from build123d import *

# Parameters (mm, degrees)
BO_ALTMA1_T                 = -1.5
KES_EKSTR_ZYON1_DEPTH       = 2
Y_KSEKLIK_EKSTR_ZYON4_DEPTH = 2
RADYUS1_R                   = 1.3
Y_KSEKLIK_EKSTR_ZYON5_DEPTH = 1.5
RADYUS2_R                   = 1
IZIM7_R                     = 2.75
KES_EKSTR_ZYON2_DEPTH       = 10
IZIM8_R                     = 1.5
KES_EKSTR_ZYON3_DEPTH       = 10
PAH1_SIZE                   = 1.656848502
PAH1_SIZE_2                 = 1.6


# Some blends are built 0.0001 mm under size
with BuildPart() as part:
    # Çizim3 → Loft4 section 0
    with BuildSketch(Plane(origin=(0, 20, 0), x_dir=(1, 0, 0), z_dir=(0, 1, 0))):
        with BuildLine():
            Line((-40, 18), (40, 18))
            Line((40, 18), (40, -18))
            Line((40, -18), (-40, -18))
            Line((-40, -18), (-40, 18))
        make_face()
    # Çizim1 → Loft4 section 1
    with BuildSketch(Plane(origin=(0, 0, 0), x_dir=(1, 0, 0), z_dir=(0, 1, 0))):
        with BuildLine():
            Line((-47.5, 25), (47.5, 25))
            Line((47.5, 25), (47.5, -25))
            Line((47.5, -25), (-47.5, -25))
            Line((-47.5, -25), (-47.5, 25))
        make_face()
    loft()

    # İç Boşaltma1
    bo_altma1_openings = [part.faces().sort_by_distance(p)[0] for p in [
        (0, 0, 0),
    ]]
    offset(amount=BO_ALTMA1_T, openings=bo_altma1_openings, kind=Kind.INTERSECTION)

    # Çizim4 → Kes-Ekstrüzyon1 (cut)
    with BuildSketch(Plane(origin=(0, 20, 0), x_dir=(1, 0, 0), z_dir=(0, 1, 0))):
        with BuildLine():
            Line((-17.459780383, 9.572622818), (-4.814835579, 9.572622818))
            ThreePointArc((-4.814835579, 9.572622818), (4.757787239, 0), (-4.814835579, -9.572622818))
            Line((-4.814835579, -9.572622818), (-17.459780383, -9.572622818))
            ThreePointArc((-17.459780383, -9.572622818), (-27.032403201, 0), (-17.459780383, 9.572622818))
        make_face()
    extrude(amount=-KES_EKSTR_ZYON1_DEPTH, mode=Mode.SUBTRACT)

    # Çizim5 → Yükseklik-Ekstrüzyon4 (add)
    with BuildSketch(Plane(origin=(0, 7.299574586, -20.855927387), x_dir=(1, 0, 0), z_dir=(0, -0.33035042472810616, 0.9438583563660173))):
        Polygon((-21.117307497, 9.666637975), (-39.739182442, 9.666637975), (-40.270102767, 8.166637975), (-21.117307497, 8.166637975), align=None)
    extrude(amount=Y_KSEKLIK_EKSTR_ZYON4_DEPTH)

    # Radyus1
    # the kernel refuses this fillet: 1.3 mm, written as the material it takes off along each edge
    with BuildSketch(Plane(origin=(-43.520102767, 14.347023232, -16.270358351), x_dir=(0, 0.3303504247281054, -0.9438583563660177), z_dir=(1, 0, 0))) as radyus1_piece_1_section:
        with BuildLine():
            CenterArc((RADYUS1_R, RADYUS1_R), RADYUS1_R, 180, 90)
            Line((0, RADYUS1_R), (0, 0))
            Line((0, 0), (RADYUS1_R, 0))
        make_face()
    radyus1_piece_1 = extrude(amount=25.65279527, mode=Mode.PRIVATE)
    radyus1_piece_1 = split(radyus1_piece_1, bisect_by=Plane(origin=(-39.107264326, 17.544066892, -15.459731471), z_dir=(0.942692407816345, -0.3149306484909819, -0.11022572697184368)), keep=Keep.TOP, mode=Mode.PRIVATE)
    add(radyus1_piece_1, mode=Mode.SUBTRACT)
    with BuildSketch(Plane(origin=(-17.867307497, 15.762810767, -15.774832714), x_dir=(0, 0.33035042472810655, -0.9438583563660172), z_dir=(-1, 0, 0))) as radyus1_piece_2_section:
        with BuildLine():
            CenterArc((RADYUS1_R, RADYUS1_R), RADYUS1_R, 180, 90)
            Line((0, RADYUS1_R), (0, 0))
            Line((0, 0), (RADYUS1_R, 0))
        make_face()
    radyus1_piece_2 = extrude(amount=25.121874944, mode=Mode.PRIVATE)
    radyus1_piece_2 = split(radyus1_piece_2, bisect_by=Plane(origin=(-38.800018931, 18.36295512, -15.171732463), z_dir=(0.942692407816345, -0.3149306484909819, -0.11022572697184368)), keep=Keep.TOP, mode=Mode.PRIVATE)
    add(radyus1_piece_2, mode=Mode.SUBTRACT)

    # Çizim6 → Yükseklik-Ekstrüzyon5 (add)
    with BuildSketch(Plane(origin=(0, 7.299574586, 20.855927387), x_dir=(-1, 0, 0), z_dir=(0, -0.3303504247281064, -0.9438583563660174))):
        Polygon((39.739182442, 9.666637975), (-7.605280372, 9.666637975), (-7.605280372, 7.666637975), (40.447076209, 7.666637975), align=None)
    extrude(amount=Y_KSEKLIK_EKSTR_ZYON5_DEPTH)

    # Radyus2
    radyus2_edges = [part.edges().sort_by_distance(p)[0] for p in [
        (-16.420897918, 14.040269266, 16.907462742),
        (-16.066951035, 15.927985979, 16.246761892),
    ]]
    fillet(radyus2_edges, radius=RADYUS2_R - 0.0001)  # a hair under: the kernel refuses the full size

    # Çizim7 → Kes-Ekstrüzyon2 (cut)
    with BuildSketch(Plane(origin=(0, 20, 0), x_dir=(1, 0, 0), z_dir=(0, 1, 0))):
        with Locations(Location((29.850184799, 0, 0), (0, 0, 270))):
            Circle(IZIM7_R)
    extrude(amount=-KES_EKSTR_ZYON2_DEPTH, mode=Mode.SUBTRACT)

    # Çizim8 → Kes-Ekstrüzyon3 (cut)
    with BuildSketch(Plane(origin=(0, 20, 0), x_dir=(1, 0, 0), z_dir=(0, 1, 0))):
        with Locations(Location((-33.057672649, 12.71180558, 0), (0, 0, 270))):
            Circle(IZIM8_R)
        with Locations(Location((33.057672649, 12.71180558, 0), (0, 0, 270))):
            Circle(IZIM8_R)
        with Locations(Location((33.057672649, -12.71180558, 0), (0, 0, 270))):
            Circle(IZIM8_R)
        with Locations(Location((-33.057672649, -12.71180558, 0), (0, 0, 270))):
            Circle(IZIM8_R)
    extrude(amount=-KES_EKSTR_ZYON3_DEPTH, mode=Mode.SUBTRACT)

    # Pah1
    # the kernel refuses this chamfer: 1.656848502, 1.6 mm, written as the material it takes off along each edge
    with BuildSketch(Plane(origin=(33.057672649, 18.5, -12.71180558), x_dir=(0, 0, 1), z_dir=(-1, 0, 0))) as pah1_piece_1:
        Polygon((1.5 + PAH1_SIZE, 0), (1.5, PAH1_SIZE_2), (1.5, 0), align=None)
    revolve(axis=Axis((33.057672649, 18.5, -12.71180558), (0, 1, 0)), mode=Mode.SUBTRACT)
    with BuildSketch(Plane(origin=(-33.057672649, 18.5, -12.71180558), x_dir=(0, 0, 1), z_dir=(-1, 0, 0))) as pah1_piece_2:
        Polygon((1.5 + PAH1_SIZE, 0), (1.5, PAH1_SIZE_2), (1.5, 0), align=None)
    revolve(axis=Axis((-33.057672649, 18.5, -12.71180558), (0, 1, 0)), mode=Mode.SUBTRACT)
    with BuildSketch(Plane(origin=(33.057672649, 18.5, 12.71180558), x_dir=(0, 0, 1), z_dir=(-1, 0, 0))) as pah1_piece_3:
        Polygon((1.5 + PAH1_SIZE, 0), (1.5, PAH1_SIZE_2), (1.5, 0), align=None)
    revolve(axis=Axis((33.057672649, 18.5, 12.71180558), (0, 1, 0)), mode=Mode.SUBTRACT)
    with BuildSketch(Plane(origin=(-33.057672649, 18.5, 12.71180558), x_dir=(0, 0, 1), z_dir=(-1, 0, 0))) as pah1_piece_4:
        Polygon((1.5 + PAH1_SIZE, 0), (1.5, PAH1_SIZE_2), (1.5, 0), align=None)
    revolve(axis=Axis((-33.057672649, 18.5, 12.71180558), (0, 1, 0)), mode=Mode.SUBTRACT)


solid = part.part
The listing builds one solid part. Answer for the finished solid, in the listing's coordinates (mm). A direction names the side the tool comes from. Give positions to 0.01 mm unless a question says otherwise; leave off trailing zeros.
Item 1: A cutting plane is placed at A-A (z = 0). Give the number of separate pieces and of enclosed holes in the cut face, then the cut area to 3 significant figures.
Derived:
separate pieces: 3
enclosed holes: 0
area: 124 mm2
Item 2: Each of these flat-tipped pins is pushed along its axis until it touches: pin 1 Ø2 at (x, y) = (-12, 9.5) entering from +Z (3 decimals); pin 2 Ø12 at (y, z) = (15, 12.5) entering from -X (3 decimals); pin 3 Ø1 at (x, y) = (19.5, 4) entering from +Z (3 decimals); pin 4 Ø10 at (x, z) = (-10, -1) entering from -Y. Where does it stop, or does it pass through?
Derived:
pin 1: stops at z = 22.025
pin 2: stops at x = -44.125
pin 3: stops at z = 23.775
pin 4: passes through
Item 3: A tool of negligible diameter and unlimited length cuts with its end or side. For faces 1 (the cylindrical face through (4.755, 19.26, -0.21)), 2 (the flat face through (9, 20, 3)), 3 (the flat face through (7.605, 15, 17)), from which of +Z, -Z, +X, -X, +Y, -Y can it reach the whole face along a straight path? Write none if from no direction.
Derived:
face 1: +Y, -Y
face 2: +Z, -Z, +X, -X, +Y
face 3: -Y
Item 4: Determine the mould class of faces 4 (the flat face through (-4, 0, 24)), 5 (the flat face through (42.48, 9.12, -0.33)) for opening direction Z: +Z half, -Z half, draft (parallel to the pull), parting line (faces both ways), or undercut.
Derived:
face 4: draft
face 5: undercut
Item 5: Find the intervals of material crossed by line 1 along X through (y, z) = (19.05, 0); line 2 along X through (y, z) = (19.4, 0) (3 decimals); line 3 along Y through (x, z) = (27.5, -10), in increasing order.
Derived:
line 1: x = -40.36 to -27.03, 4.76 to 27.1, 32.6 to 40.36
line 2: x = -40.225 to -27.032, 4.758 to 27.1, 32.6 to 40.225
line 3: y = 18.5 to 20
